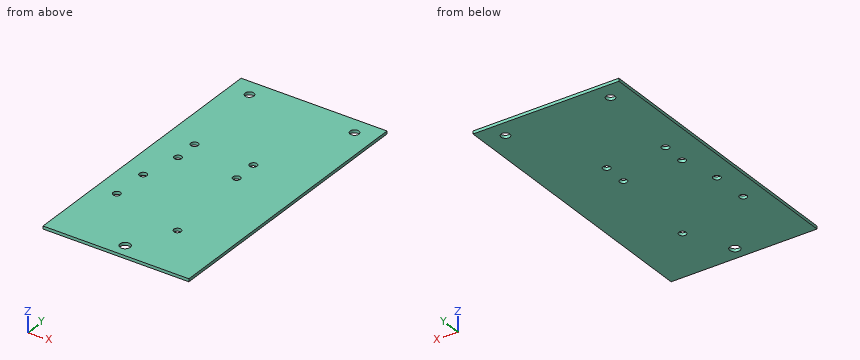
```python
from build123d import *

# Parameters (mm, degrees)
F0_W     = 100
F0_H     = 30
F0_R     = 3.5
F0_H_2   = 100
F0_R_2   = 2.5
F0_H_3   = 65
F0_R_3   = 3
F1_DEPTH = 2


with BuildPart() as f1:
    # F0 (on Top) → F1 (new body)
    with BuildSketch(Plane.XY):
        with Locations((50, 11.390658)):
            Rectangle(F0_W, F0_H)
        with Locations((50, 5.390658)):
            Circle(F0_R, mode=Mode.SUBTRACT)
        with Locations((50, 76.390658)):
            Rectangle(F0_W, F0_H_2)
        with Locations((14.045889, 48.890658)):
            Circle(F0_R_2, mode=Mode.SUBTRACT)
        with Locations((14.371501, 74.288571)):
            Circle(F0_R_2, mode=Mode.SUBTRACT)
        with Locations((64.845889, 35.633259)):
            Circle(F0_R_2, mode=Mode.SUBTRACT)
        with Locations((19.840248, 100.720075)):
            Circle(F0_R_2, mode=Mode.SUBTRACT)
        with Locations((19.357387, 117.720075)):
            Circle(F0_R_2, mode=Mode.SUBTRACT)
        with Locations((59.722181, 101.20294)):
            Circle(F0_R_2, mode=Mode.SUBTRACT)
        with Locations((59.357387, 118.20294)):
            Circle(F0_R_2, mode=Mode.SUBTRACT)
        with Locations((50, 158.890658)):
            Rectangle(F0_W, F0_H_3)
        with Locations((14, 179.526627)):
            Circle(F0_R_3, mode=Mode.SUBTRACT)
        with Locations((86, 179.526627)):
            Circle(F0_R_3, mode=Mode.SUBTRACT)
    extrude(amount=F1_DEPTH)


solid = f1.part
```
Can you work these out from the model? Positions are in its coordinate system, mm. Coordinates: 2 decimals unless noted, no trailing zeros. Loops run counter-clockwise (first coordinate to the right, second up) from the corner with the lowest first, then second, coordinate; pieces in that order, holes last. Notation, with made-up numbers: (7.25, 86) - (41.25, 86) arc R11 ccw to (41.25, 102) - close; hole circle Ø11 at (39, -38). An arc over 180 degrees is marked (long way). Answer as CSV lines item,"result". Start each with the question number.
1) Suppose I cut it at A-A (x = 50). Please give me the cut outline in (y, z), plus the area to 3 significant figures.
2) Suppose I cut it at C-C (x = 86). Please give me the cut outline in (y, z), plus the area to 3 significant figures.
3) I need wall thicknesses on line 1 (Y direction, x = 14, z = 1.2); line 2 (Y direction, x = 58.5, z = 1.8); line 3 (X direction, y = 99.5, z = 1.35). Which ranges of each line are inside material? Lowest first, please. Write a range as from..to.
4) Suppose I cut it at B-B (x = 14). Please give me the cut outline in (y, z).
Check result:
1,outline,"(-3.61, 0) - (1.89, 0) - (1.89, 2) - (-3.61, 2) - close; (8.89, 0) - (191.39, 0) - (191.39, 2) - (8.89, 2) - close"
1,area,"376 mm²"
2,outline,"(-3.61, 0) - (176.53, 0) - (176.53, 2) - (-3.61, 2) - close; (182.53, 0) - (191.39, 0) - (191.39, 2) - (182.53, 2) - close"
2,area,"378 mm²"
3,line 1,"y = -3.61..46.39, 51.39..71.82, 76.76..176.53, 182.53..191.39"
3,line 2,"y = -3.61..99.02, 103.38..115.85, 120.55..191.39"
3,line 3,"x = 0..17.66, 22.02..57.89, 61.55..100"
4,outline,"(-3.61, 0) - (46.39, 0) - (46.39, 2) - (-3.61, 2) - close; (51.39, 0) - (71.82, 0) - (71.82, 2) - (51.39, 2) - close; (76.76, 0) - (176.53, 0) - (176.53, 2) - (76.76, 2) - close; (182.53, 0) - (191.39, 0) - (191.39, 2) - (182.53, 2) - close"
